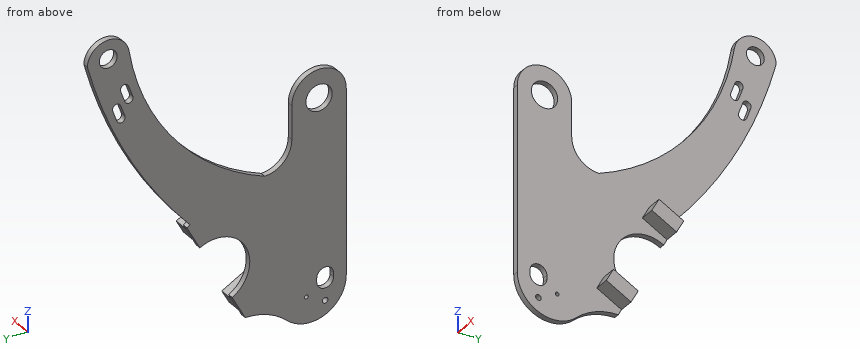
```python
from build123d import *

# Parameters (mm, degrees)
SKETCH1_R           = 1.5
SKETCH1_R_2         = 1
SKETCH1_R_3         = 7
SKETCH1_R_4         = 4.75
BOSS_EXTRUDE1_DEPTH = 3
BOSS_EXTRUDE2_DEPTH = 8


with BuildPart() as part:
    # Sketch1 → Boss-Extrude1 (new body)
    with BuildSketch(Plane(origin=(0, 0, 0), x_dir=(0, 0, -1), z_dir=(1, 0, 0))):
        with BuildLine():
            Line((-49.159345461, 0), (49.159345461, 0))
            ThreePointArc((49.159345461, 0), (66.340654539, 11.242329364), (62.91845049, 31.487720707))
            ThreePointArc((62.91845049, 31.487720707), (56.432557087, 41.829379484), (54.166473214, 53.824444444))
            Line((54.166473214, 53.824444444), (41.340654539, 60.8))
            ThreePointArc((41.340654539, 60.8), (16.928001378, 53.587346839), (9.715348216, 78))
            Line((9.715348216, 78), (-3.110470459, 84.975555556))
            Line((-3.110470459, 84.975555556), (-4.066026015, 83.218594093))
            ThreePointArc((-4.066026015, 83.218594093), (-51.126972403, 116.596460909), (-104.705915866, 138))
            ThreePointArc((-104.705915866, 138), (-115.275757126, 127.38864025), (-105.87300769, 115.730561375))
            ThreePointArc((-105.87300769, 115.730561375), (-51.706077225, 91.471635272), (-16.759345461, 43.5))
            ThreePointArc((-16.759345461, 43.5), (-21.006297134, 33.246951673), (-31.259345461, 29))
            Line((-31.259345461, 29), (-49.159345461, 29))
            ThreePointArc((-49.159345461, 29), (-63.659345461, 14.5), (-49.159345461, 0))
        make_face()
        with Locations((58.840654539, 11.242329364)):
            Circle(SKETCH1_R, mode=Mode.SUBTRACT)
        with Locations((53.840654539, 21.242329364)):
            Circle(SKETCH1_R_2, mode=Mode.SUBTRACT)
        with Locations((-48.659345461, 14.5)):
            Circle(SKETCH1_R_3, mode=Mode.SUBTRACT)
        with Locations((-105.289461778, 126.865280687)):
            Circle(SKETCH1_R_4, mode=Mode.SUBTRACT)
        with BuildLine():
            Line((45.840654539, 15.742329364), (47.840654539, 15.742329364))
            ThreePointArc((47.840654539, 15.742329364), (52.340654539, 11.242329364), (47.840654539, 6.742329364))
            Line((47.840654539, 6.742329364), (45.840654539, 6.742329364))
            ThreePointArc((45.840654539, 6.742329364), (41.340654539, 11.242329364), (45.840654539, 15.742329364))
        make_face(mode=Mode.SUBTRACT)
        with BuildLine():
            Line((-86.096000708, 120.210043762), (-79.987998673, 117.98691283))
            ThreePointArc((-79.987998673, 117.98691283), (-78.643235599, 115.103059111), (-81.527089318, 113.758296037))
            Line((-81.527089318, 113.758296037), (-87.635091353, 115.981426968))
            ThreePointArc((-87.635091353, 115.981426968), (-88.979854428, 118.865280687), (-86.096000708, 120.210043762))
        make_face(mode=Mode.SUBTRACT)
        with BuildLine():
            Line((-77.104144954, 124.438660555), (-70.996142919, 122.215529624))
            ThreePointArc((-70.996142919, 122.215529624), (-69.651379845, 119.331675904), (-72.535233564, 117.98691283))
            Line((-72.535233564, 117.98691283), (-78.643235599, 120.210043762))
            ThreePointArc((-78.643235599, 120.210043762), (-79.987998673, 123.093897481), (-77.104144954, 124.438660555))
        make_face(mode=Mode.SUBTRACT)
    extrude(amount=BOSS_EXTRUDE1_DEPTH)

    # Sketch2 → Boss-Extrude2 (add)
    with BuildSketch(Plane(origin=(3, 0, 0), x_dir=(0, 0, -1), z_dir=(1, 0, 0))):
        Polygon((43.976096732, 59.366666667), (51.003942582, 55.544444444), (43.837275915, 42.367233477), (36.809430066, 46.189455699), align=None)
        Polygon((-0.650724412, 83.637777778), (6.377121438, 79.815555556), (-0.789545229, 66.638344588), (-7.817391078, 70.46056681), align=None)
    extrude(amount=BOSS_EXTRUDE2_DEPTH)


solid = part.part
```
Here's how the part is built. I have some questions about the finished solid (model axes, mm). Give positions to 0.01 mm unless a question says otherwise; leave off trailing zeros. Order: outer loops, then holes, each group sorted by start corner. A loop starts at its lowest first (then second) coordinate and runs counter-clockwise, first axis right, second up. Notation, with made-up numbers: (53.25, 27.25) -> (99.25, 27.25) arc R24 cw to (99.25, 47.25) -> close; hole circle Ø2 at (19, 62). An arc over 180 degrees is marked (long way). Use CSV: the item, a comma, the result in double quotes. Start each with the question number.
Item 1: If I drill on probe 1 along Y at (x, z) = (1.5, 46); probe 2 along X at (y, z) = (24, 44); probe 3 along Z at (x, y) = (2.75, 59), over which ranges is the centre line in solid material (lowest first)? Write a range as [from, to].
Item 2: Suppose I cut it at A-A (x = 5). List the corners of the cut face in (y, z) for me.
Item 3: I'm going to push flat-ended pins straight in: P1, Ø0.6, axis at x = 1, z = -46.5, coming from the +Y side; P2, Ø5, axis at y = 23, z = 29, coming from the +X side; P3, Ø1.5, axis at x = 1, z = 43.5, coming from the +Y side; P4, Ø1.2, axis at y = 21.24, z = -53.84, coming from the +X side. Where does each tip first touch, or does it pass through?
Item 4: Suppose I cut it at B-B (z = 60). List the corners of the cut face in (x, y) for me.
Item 5: Suppose I cut it at C-C (y = 37.5). List the corners of the cut face in (x, z) for me, and give its area (3 significant figures).
Answer block:
1,probe 1,"y = [0, 8.02], [20.98, 29], [86.53, 113.73]"
1,probe 2,"x = [0, 3]"
1,probe 3,"z = [-44.65, -40.22], [-10.84, 24.13]"
2,outline,"(42.37, -43.84) -> (55.54, -51) -> (59.37, -43.98) -> (46.19, -36.81) -> close; (66.64, 0.79) -> (79.82, -6.38) -> (83.64, 0.65) -> (70.46, 7.82) -> close"
3,P1,"stops at y = 58.16"
3,P2,"stops at x = 3"
3,P3,"stops at y = 112.71"
3,P4,"passes through"
4,outline,"(0, 4.87) -> (3, 4.87) -> (3, 24.13) -> (0, 24.13) -> close; (0, 97.6) -> (3, 97.6) -> (3, 121.19) -> (0, 121.19) -> close"
5,outline,"(0, -58.51) -> (3, -58.51) -> (3, 18.06) -> (0, 18.06) -> close"
5,area,"230 mm^2"
